from build123d import *

# Parameters (mm, degrees)
SKETCH1_W                        = 60
SKETCH1_H                        = 125
BOSS_EXTRUDE1_DEPTH              = 10
SKETCH2_R                        = 9.5
BOSS_EXTRUDE2_DEPTH              = 25
CUT_EXTRUDE1_REACH               = 164.114
SKETCH3_R                        = 2.75
M10X1_0_TAPPED_HOLE1_D           = 9
M14X1_5_TAPPED_HOLE1_D           = 12.5
M14X1_5_TAPPED_HOLE1_CSINK_D     = 14.05
M14X1_5_TAPPED_HOLE1_CSINK_ANGLE = 90
FILLET1_R                        = 10


with BuildPart() as part:
    # Sketch1 → Boss-Extrude1 (new body)
    with BuildSketch(Plane(origin=(0, 0, 0), x_dir=(1, 0, 0), z_dir=(0, 1, 0))):
        with Locations((30, 62.5)):
            Rectangle(SKETCH1_W, SKETCH1_H)
    extrude(amount=BOSS_EXTRUDE1_DEPTH)

    # Sketch2 → Boss-Extrude2 (add)
    with BuildSketch(Plane(origin=(0, 0, -125), x_dir=(-1, 0, 0), z_dir=(0, 0, -1))):
        with BuildLine():
            Line((-60, 10), (0, 10))
            Line((0, 10), (0, 64))
            ThreePointArc((0, 64), (-30, 94), (-60, 64))
            Line((-60, 64), (-60, 10))
        make_face()
        with Locations((-30, 64)):
            Circle(SKETCH2_R, mode=Mode.SUBTRACT)
    extrude(amount=-BOSS_EXTRUDE2_DEPTH)

    # Sketch3 → Cut-Extrude1 (cut, up to next)
    with BuildSketch(Plane(origin=(0, 10, 0), x_dir=(1, 0, 0), z_dir=(0, 1, 0)), mode=Mode.PRIVATE) as cut_extrude1_sk1:
        with Locations(Location((30, 50, 0), (0, 0, 270))):
            Circle(SKETCH3_R)
    cut_extrude1_tool1 = extrude(cut_extrude1_sk1.sketch, amount=-CUT_EXTRUDE1_REACH, mode=Mode.PRIVATE) & part.part
    add(cut_extrude1_tool1.solids().sort_by_distance((30, 10, -50))[0], mode=Mode.SUBTRACT)

    # M10x1.0 Tapped Hole1 (through all)
    with Locations(Plane(origin=(0, 10, 0), x_dir=(1, 0, 0), z_dir=(0, 1, 0))):
        with Locations((30, 75)):
            Hole(M10X1_0_TAPPED_HOLE1_D / 2)

    # M14x1.5 Tapped Hole1 (through all)
    with Locations(Plane(origin=(0, 10, 0), x_dir=(1, 0, 0), z_dir=(0, 1, 0))):
        with Locations((30, 25)):
            CounterSinkHole(M14X1_5_TAPPED_HOLE1_D / 2, M14X1_5_TAPPED_HOLE1_CSINK_D / 2, counter_sink_angle=M14X1_5_TAPPED_HOLE1_CSINK_ANGLE)

    # Fillet1
    fillet1_edges = [part.edges().sort_by_distance(p)[0] for p in [
        (30, 10, -100),
    ]]
    fillet(fillet1_edges, radius=FILLET1_R)


solid = part.part
Can you work these out from the model? Positions are in its coordinate system, mm. A direction names the side the tool comes from. Coordinates: 2 decimals unless noted, no trailing zeros. Write each loop counter-clockwise with the first axis right and the second up, starting at its lowest first coordinate (ties: lowest second). Pieces come first, ordered by that corner, then holes. Notation, with made-up numbers: M 1.25,-31 L 8.25,-31 A20 ccw 8.25,-23 Z; hole C -16,39.5 d1. An arc over 180 degrees is marked long. Use one line per item in the form item = value.
Q1. We'd pull the mould along Z, two halves only. Please class faces 1 (the cylindrical face through (27.581, 4.93, -78.794)), 2 (the cylindrical face through (31.355, 4.548, -18.899)), 3 (the flat face through (30, 48, -125)), 4 (the cylindrical face through (31.24, 73.42, -112.68)): +Z half, -Z half, draft (parallel to the pull), parting line (faces both ways), or undercut.
Model answer:
face_1 = undercut
face_2 = undercut
face_3 = -Z half
face_4 = draft
Q2. If we section it at D-D (x = 6): Write out the boundary of the cut face in (y, z), then the cut area to 3 significant figures.
Model answer:
outline = M 0,-125 L 82,-125 L 82,-100 L 20,-100 A10 cw 10,-90 L 10,0 L 0,0 Z
area = 3,070 mm^2
Q3. For faces 5 (the flat face through (30, 10, -46)), 6 (the flat face through (30, 5, 0)), which set-ups out of +Z, -Z, +X, -X, +Y, -Y let a thin tool reach every point of the face, with its end or its side?
Model answer:
face_5 = +Z, +X, -X, +Y
face_6 = +Z, +X, -X, +Y, -Y
Q4. If we section it at A-A (z = -50): Write out the boundary of the cut face in (x, y), then the cut area to 3 significant figures.
Model answer:
outline = M 0,0 L 27.25,0 L 27.25,10 L 0,10 Z; M 32.75,0 L 60,0 L 60,10 L 32.75,10 Z
area = 545 mm^2
Q5. If we section it at C-C (y = 61): Write out the boundary of the cut face in (x, z).
Model answer:
outline = M 0,-125 L 20.99,-125 L 20.99,-100 L 0,-100 Z; M 39.01,-125 L 60,-125 L 60,-100 L 39.01,-100 Z
Q6. If we section it at B-B (x = 30): Write out the boundary of the cut face in (y, z) (3 decimals), then the cut area to 3 significant figures.
Model answer:
outline = M 0,-125 L 54.5,-125 L 54.5,-100 L 20,-100 A10 cw 10,-90 L 10,-79.5 L 0,-79.5 Z; M 0,-70.5 L 10,-70.5 L 10,-52.75 L 0,-52.75 Z; M 0,-47.25 L 10,-47.25 L 10,-32.025 L 9.225,-31.25 L 0,-31.25 Z; M 0,-18.75 L 9.225,-18.75 L 10,-17.975 L 10,0 L 0,0 Z; M 73.5,-125 L 94,-125 L 94,-100 L 73.5,-100 Z
area = 2,630 mm^2
Q7. I need wall thicknesses on line 1 along X through (y, z) = (3.75, -50); line 2 along X through (y, z) = (5, -25); line 3 along Y through (x, z) = (30, -117). Which ranges of each line are inside material? Lowest first, please. Write a range as from..to.
Model answer:
line_1 = 0..27.25, 32.75..60
line_2 = 0..23.75, 36.25..60
line_3 = 0..54.5, 73.5..94
Q8. For P1, Ø9, axis at x = 30, z = -50, coming from the +Y side; P2, Ø2, axis at x = 48.5, z = -76.5, coming from the -Y side; P3, Ø8, axis at x = 24, y = 47.5, coming from the +Z side, each with a flat end and sliding along its axis, tell me the tip position at first contact or that it passes through.
Model answer:
P1 = 10
P2 = 0
P3 = -100
